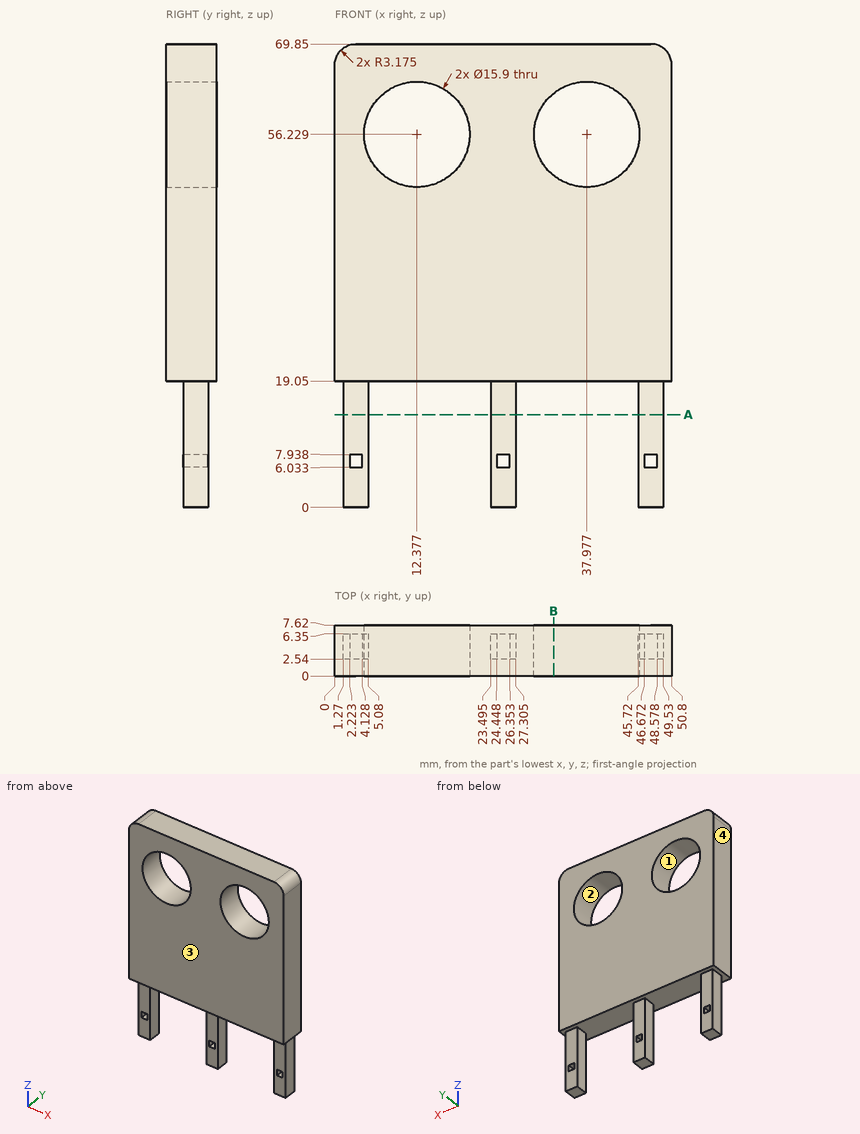
For this review, use the dimensioned drawing (mm, ordinates from the lowest corner) and the shaded views. Round coordinates to 2 decimals unless told otherwise and drop trailing zeros. Write each loop counter-clockwise with the first axis right and the second up, starting at its lowest first coordinate (ties: lowest second). Pieces come first, ordered by that corner, then holes. Notation, with made-up numbers: (39, -16.5) -> (56, -16.5) arc R10 ccw to (56, -1.5) -> close; hole circle Ø6 at (-9.75, -6.5). An arc over 180 degrees is marked (long way). Answer in a Markdown table with one row per item.
Q1. Draft analysis for pull direction X (two halves, no side actions). For the marked faces 1, 2, 3 and 4, state which applies: +X half, -X half, draft (parallel to the pull), parting line (faces both ways), or undercut.
The answers:
| item | result |
|---|---|
| face 1 | undercut |
| face 2 | undercut |
| face 3 | draft |
| face 4 | -X half |
Q2. Take a section at A-A, the plane z = 14. Count the separate pieces of the cut face and the enclosed holes in it.
The answers:
| item | result |
|---|---|
| separate pieces | 3 |
| enclosed holes | 0 |
Q3. Take a section at B-B, the plane x = 33. State the section outline as (y, z) points, then the cut area to 3 significant figures.
The answers:
| item | result |
|---|---|
| outline | (0, 19.05) -> (7.62, 19.05) -> (7.62, 50.03) -> (0, 50.03) -> close; (0, 62.43) -> (7.62, 62.43) -> (7.62, 69.85) -> (0, 69.85) -> close |
| area | 293 mm² |
Q4. To check wall thickness, follow L1, parallel to X at y = 3, z = 4 (1 decimal); L2, parallel to X at y = 2.5, z = 60.5; L3, parallel to Y at x = 24.5, z = 4.5. State the ranges of each line that lie inside material, in increasing order. Write a range as [from, to].
The answers:
| item | result |
|---|---|
| L1 | [1.3, 5.1], [23.5, 27.3], [45.7, 49.5] |
| L2 | [0, 5.67], [19.08, 31.27], [44.68, 50.8] |
| L3 | [2.54, 6.35] |
Q5. Clearance check with flat-ended pins moving along their axes: pin 1 Ø6 at (x, z) = (8.5, 15) entering from +Y; pin 2 Ø2 at (x, y) = (41, 1.5) entering from -Z; pin 3 Ø1.9 at (x, z) = (2.5, 6.5) entering from -Y; pin 4 Ø0.6 at (y, z) = (4.5, 7) entering from -X. State where each tip first meets the part, or that it passes through.
The answers:
| item | result |
|---|---|
| pin 1 | through |
| pin 2 | z = 19.05 |
| pin 3 | y = 2.54 |
| pin 4 | x = 1.27 |
